from build123d import *

# Parameters (mm, degrees)
F0_W     = 317.5
F0_H     = 431.8
F1_DEPTH = 279.4
F2_R     = 6.35
F3_DEPTH = 12.7
F4_R     = 6.35
F5_DEPTH = 12.7


with BuildPart() as f1:
    # F0 (on Top) → F1 (new body)
    with BuildSketch(Plane.XY):
        with Locations((-158.75, 215.9)):
            Rectangle(F0_W, F0_H)
    extrude(amount=F1_DEPTH)

    # F2 (on face) → F3 (join)
    with BuildSketch(Plane(origin=(0, 431.8, 0), x_dir=(-1, 0, 0), z_dir=(0, 1, 0))):
        with Locations((158.75, 6.35)):
            Circle(F2_R)
    extrude(amount=F3_DEPTH)

    # F4 (on face) → F5 (join)
    with BuildSketch(Plane.XZ):
        with BuildLine():
            ThreePointArc((-298.45, 273.05), (-292.1, 266.7), (-285.75, 273.05))
            ThreePointArc((-285.75, 273.05), (-292.1, 279.4), (-298.45, 273.05))
        make_face()
        with Locations((-25.4, 273.05)):
            Circle(F4_R)
    extrude(amount=F5_DEPTH)


solid = f1.part
Could you check a few things on this model? Use its own coordinates, in mm. A direction names the side the tool comes from. Give positions to 0.01 mm unless a question says otherwise; leave off trailing zeros. Loops run counter-clockwise (first coordinate to the right, second up) from the corner with the lowest first, then second, coordinate; pieces in that order, holes last. Notation, with made-up numbers: (14.25, 67) -> (37.25, 67) arc R7 cw to (37.25, 74) -> close; hole circle Ø2 at (-20.5, 83.25). An arc over 180 degrees is marked (long way). Return JSON: item names as keys, results as strings.
Item 1: I need wall thicknesses on L1, parallel to Y at x = -36, z = 13. Which ranges of the line are inside material? Lowest first, please. Write a range as from..to.
Geometry results:
{"L1": "y = 0..431.8"}
Item 2: If we section it at A-A on z = 273.05: List the corners of the cut face in (x, y) for me.
Geometry results:
{"outline": "(-317.5, 0) -> (-298.45, 0) -> (-298.45, -12.7) -> (-285.75, -12.7) -> (-285.75, 0) -> (-31.75, 0) -> (-31.75, -12.7) -> (-19.05, -12.7) -> (-19.05, 0) -> (0, 0) -> (0, 431.8) -> (-317.5, 431.8) -> close"}
Item 3: I'm going to push a flat-ended pin straight in: pin 1 (1 mm diameter, centred on x = -231.5, z = 123, fed in from +Y). Where does the tip first touch, or does it pass through?
Geometry results:
{"pin 1": "stops at y = 431.8"}
Item 4: If we section it at B-B on x = -188.5: List the corners of the cut face in (y, z) for me, plus the area to 3 significant figures.
Geometry results:
{"outline": "(0, 0) -> (431.8, 0) -> (431.8, 279.4) -> (0, 279.4) -> close", "area": "121,000 mm²"}
Item 5: If we section it at C-C on z = 6.35: List the corners of the cut face in (x, y) for me.
Geometry results:
{"outline": "(-317.5, 0) -> (0, 0) -> (0, 431.8) -> (-152.4, 431.8) -> (-152.4, 444.5) -> (-165.1, 444.5) -> (-165.1, 431.8) -> (-317.5, 431.8) -> close"}
Item 6: Which directions (+Z, -Z, +X, -X, +Y, -Y) give clear straight access to the entire face, cutting with the end or side of a thin tool? Please do faces 1 (the flat face through (-25, -12.7, 273)), 2 (the cylindrical face through (-297.14, -6.26, 269.19)).
Geometry results:
{"face 1": "+Z, -Z, +X, -X, -Y", "face 2": "-Y"}
Item 7: We'd pull the mould along X, two halves only. Please class faces 3 (the cylindrical face through (-26.78, -6.26, 266.85)), 4 (the cylindrical face through (-164.807, 438.061, 8.257)), 5 (the flat face through (-161, 219, 0)): +X half, -X half, draft (parallel to the pull), parting line (faces both ways), or undercut.
Geometry results:
{"face 3": "undercut", "face 4": "parting line", "face 5": "draft"}
